```python
from build123d import *

# Parameters (mm, degrees)
CHAMFER1_SIZE = 0.5


with BuildPart() as part:
    # Sketch1 → Revolve1 (revolve)
    with BuildSketch(Plane.XY):
        Polygon((4, 0), (4, 12), (7.5, 12), (7.5, 8.75), (7.15, 8.75), (7.15, 7.65), (7.5, 7.65), (7.5, 0), align=None)
    revolve(axis=Axis((0, 0, 0), (0, 1, 0)))

    # Chamfer1
    chamfer1_edges = [part.edges().sort_by_distance(p)[0] for p in [
        (-7.5, 12, 0),
    ]]
    chamfer(chamfer1_edges, length=CHAMFER1_SIZE)

    # Mirror1: part across plane


with BuildPart() as part_1:
    add(part.part)
    add(part.part.mirror(Plane(origin=(7.5, 0, 0), x_dir=(0, 0, 1), z_dir=(0, -1, 0))))


solid = part_1.part
```
Part model, mm, in its own coordinate system. A direction names the side the tool comes from. Coordinates: 2 decimals unless noted, no trailing zeros. Write each loop counter-clockwise with the first axis right and the second up, starting at its lowest first coordinate (ties: lowest second). Pieces come first, ordered by that corner, then holes.
Item 1: Slice it at C-C (y = -4.5). Write the cut outline in (x, z).
Item 2: Slice it at A-A (x = 0). Write the cut outline in (y, z), and give its area (3 significant figures).
Item 3: Which spindle directions (+Z, -Z, +X, -X, +Y, -Y) get a long thin tool onto all of the face, cutting with end or side? Do faces 1 (the face through (-0.93, 8.19, -7.09)), 2 (the face through (-7.493, 10.106, -0.33)). Say none if no direction does.
Item 4: Pin check, flat tips, straight feed: pin 1 (2 mm diameter, centred on y = -3.5, z = -4.5, fed in from +X); pin 2 (8 mm diameter, centred on x = -4.5, y = 8, fed in from +Z); pin 3 (2 mm diameter, centred on x = 4.5, y = -3.5, fed in from -Z). Stop position of each tip, or through.
Item 5: Slice it at B-B (z = 0). Write the cut outline in (x, y), and give its area (3 significant figures).
Item 6: Mould opens along Y. For faces 3 (the face through (-3, 12, 3)), 4 (the face through (-7.493, -10.106, -0.33)), 5 (the face through (-0.93, -8.19, -7.09)), 6 (the face through (-3, -12, 3)) say: released by +Y, released by -Y, zero draft, split by the parting line, or undercut.
Item 7: Probe line 1 (Z direction, x = 0, y = 5.5); line 2 (Z direction, x = 0, y = 8). List the from-to ranges inside material, lowest first.
Results found:
1. outline: circle Ø15 at (0, 0); hole circle Ø8 at (0, 0)
2. outline: (-12, -7) - (-11.5, -7.5) - (-8.75, -7.5) - (-8.75, -7.15) - (-7.65, -7.15) - (-7.65, -7.5) - (7.65, -7.5) - (7.65, -7.15) - (8.75, -7.15) - (8.75, -7.5) - (11.5, -7.5) - (12, -7) - (12, -4) - (-12, -4) - close; (-12, 4) - (12, 4) - (12, 7) - (11.5, 7.5) - (8.75, 7.5) - (8.75, 7.15) - (7.65, 7.15) - (7.65, 7.5) - (-7.65, 7.5) - (-7.65, 7.15) - (-8.75, 7.15) - (-8.75, 7.5) - (-11.5, 7.5) - (-12, 7) - close
2. area: 166 mm2
3. face 1: none
3. face 2: +Y, -Y
4. pin 1: stops at x = 6.63
4. pin 2: stops at z = 7.48
4. pin 3: stops at z = -6.63
5. outline: (-7.5, -11.5) - (-7, -12) - (-4, -12) - (-4, 12) - (-7, 12) - (-7.5, 11.5) - (-7.5, 8.75) - (-7.15, 8.75) - (-7.15, 7.65) - (-7.5, 7.65) - (-7.5, -7.65) - (-7.15, -7.65) - (-7.15, -8.75) - (-7.5, -8.75) - close; (4, -12) - (7, -12) - (7.5, -11.5) - (7.5, -8.75) - (7.15, -8.75) - (7.15, -7.65) - (7.5, -7.65) - (7.5, 7.65) - (7.15, 7.65) - (7.15, 8.75) - (7.5, 8.75) - (7.5, 11.5) - (7, 12) - (4, 12) - close
5. area: 166 mm2
6. face 3: released by +Y
6. face 4: zero draft
6. face 5: undercut
6. face 6: released by -Y
7. line 1: z = -7.5 to -4, 4 to 7.5
7. line 2: z = -7.15 to -4, 4 to 7.15
